```python
from build123d import *

# Parameters (mm, degrees)
F0_W     = 50
F0_H     = 50
F0_R     = 2
F1_DEPTH = 3
F2_D     = 4.5


# Not quite as in the source:
# - a feature names something its author has since deleted; it is built from what else it names


with BuildPart() as f1:
    # F0 (on Top) → F1 (new body)
    with BuildSketch(Plane.XY):
        with Locations((-50, -49.9732751399)):
            Rectangle(F0_W, F0_H)
        with Locations((-67.5, -67.4732751399)):
            Circle(F0_R, mode=Mode.SUBTRACT)
        with Locations((-32.5, -67.4732751399)):
            Circle(F0_R, mode=Mode.SUBTRACT)
        with Locations((-67.5, -32.4732751399)):
            Circle(F0_R, mode=Mode.SUBTRACT)
        with BuildLine():
            Line((-47.5, -40.9732751399), (-47.5, -43.4349267246))
            ThreePointArc((-47.5, -43.4349267246), (-44.2337187027, -46.0046481733), (-43, -49.9732751399))
            ThreePointArc((-43, -49.9732751399), (-53.9686269666, -55.7395564373), (-52.5, -43.4349267246))
            Line((-52.5, -43.4349267246), (-52.5, -40.9732751399))
            Line((-52.5, -40.9732751399), (-47.5, -40.9732751399))
        make_face(mode=Mode.SUBTRACT)
        with Locations((-32.5, -32.4732751399)):
            Circle(F0_R, mode=Mode.SUBTRACT)
    extrude(amount=F1_DEPTH)

    # F2 (through all)
    with Locations(Plane(origin=(0, 0, 0), x_dir=(1, 0, 0), z_dir=(0, 0, -1))):
        with Locations((-32.5, 32.4732751399), (-32.5, 67.4732751399), (-67.5, 67.4732751399), (-67.5, 32.4732751399)):
            Hole(F2_D / 2)


solid = f1.part
```
Model file for the job. Use its own axes, mm. A direction names the side the tool comes from. Give positions to 0.01 mm unless a question says otherwise; leave off trailing zeros. Order: outer loops, then holes, each group sorted by start corner. A loop starts at its lowest first (then second) coordinate and runs counter-clockwise, first axis right, second up.
1) Saw through at A-A, the plane x = -50. Write the cut outline in (y, z), then the cut area to 3 significant figures.
2) Wall check: probe 1 along Y at (x, z) = (-32.5, 1); probe 2 along Y at (x, z) = (-67, 0.3); probe 3 along X at (y, z) = (-44.5, 1.9). Give the ranges that are in metal, low to high.
3) Saw through at D-D, the plane z = 1. Write the cut outline in (x, y).
4) Saw through at C-C, the plane x = -32.5. Write the cut outline in (y, z), then the cut area to 3 significant figures.
5) Saw through at B-B, the plane y = -48. Write the cut outline in (x, z).
6) 3-axis set-ups, long thin cutter, end or side, ignore diameter. For faces 5 (the flat face through (-56, -44, 3)), 6 (the flat face through (-47.5, -42, 1)): which of +Z, -Z, +X, -X, +Y, -Y reach the whole face in a straight line?
7) Mould opens along X. For faces 1 (the flat face through (-50, -40.973, 1)), 2 (the cylindrical face through (-32.207, -69.704, 1.521)), 3 (the flat face through (-25, -50, 1)), 4 (the flat face through (-56, -44, 0)) say: +X half, -X half, draft (parallel to the pull), parting line (faces both ways), or undercut.
Computed:
1. outline: (-74.97, 0) - (-56.97, 0) - (-56.97, 3) - (-74.97, 3) - close; (-40.97, 0) - (-24.97, 0) - (-24.97, 3) - (-40.97, 3) - close
1. area: 102 mm2
2. probe 1: y = -74.97 to -69.72, -65.22 to -34.72, -30.22 to -24.97
2. probe 2: y = -74.97 to -69.67, -65.28 to -34.67, -30.28 to -24.97
2. probe 3: x = -75 to -54.36, -45.64 to -25
3. outline: (-75, -74.97) - (-25, -74.97) - (-25, -24.97) - (-75, -24.97) - close; hole circle Ø4.5 at (-67.5, -67.47); hole circle Ø4.5 at (-67.5, -32.47); hole (-52.5, -43.43) arc R7 ccw (long way) to (-47.5, -43.43) - (-47.5, -40.97) - (-52.5, -40.97) - close; hole circle Ø4.5 at (-32.5, -67.47); hole circle Ø4.5 at (-32.5, -32.47)
4. outline: (-74.97, 0) - (-69.72, 0) - (-69.72, 3) - (-74.97, 3) - close; (-65.22, 0) - (-34.72, 0) - (-34.72, 3) - (-65.22, 3) - close; (-30.22, 0) - (-24.97, 0) - (-24.97, 3) - (-30.22, 3) - close
4. area: 123 mm2
5. outline: (-75, 0) - (-56.72, 0) - (-56.72, 3) - (-75, 3) - close; (-43.28, 0) - (-25, 0) - (-25, 3) - (-43.28, 3) - close
6. face 5: +Z, +X, -X, +Y, -Y
6. face 6: +Z, -Z
7. face 1: undercut
7. face 2: undercut
7. face 3: +X half
7. face 4: draft
